from build123d import *

# Parameters (mm, degrees)
BOSS_EXTRUDE1_DEPTH = 10
SKETCH2_R           = 10.45
CUT_EXTRUDE1_DEPTH  = 7
SKETCH3_R           = 6.5
CUT_EXTRUDE2_DEPTH  = 24.087280048


with BuildPart() as part:
    # Sketch1 → Boss-Extrude1 (new body)
    with BuildSketch(Plane.YZ):
        with BuildLine():
            Line((-12.65, 0), (-12.65, 18))
            Line((-12.65, 18), (12.65, 18))
            Line((12.65, 18), (12.65, 0))
            ThreePointArc((12.65, 0), (0, -12.65), (-12.65, 0))
        make_face()
    extrude(amount=BOSS_EXTRUDE1_DEPTH)

    # Sketch2 → Cut-Extrude1 (cut)
    with BuildSketch(Plane.YZ.offset(10)):
        with Locations(Location((0, 0, 0), (0, 0, 270))):
            Circle(SKETCH2_R)
    extrude(amount=-CUT_EXTRUDE1_DEPTH, mode=Mode.SUBTRACT)

    # Sketch3 → Cut-Extrude2 (cut, through all)
    with BuildSketch(Plane.YZ.offset(3)):
        with Locations(Location((0, 0, 0), (0, 0, 270))):
            Circle(SKETCH3_R)
    extrude(amount=-CUT_EXTRUDE2_DEPTH, mode=Mode.SUBTRACT)


solid = part.part
The listing builds one solid part. Answer for the finished solid, in the listing's coordinates (mm). A direction names the side the tool comes from. Give positions to 0.01 mm unless a question says otherwise; leave off trailing zeros. Write each loop counter-clockwise with the first axis right and the second up, starting at its lowest first coordinate (ties: lowest second). Pieces come first, ordered by that corner, then holes.
Item 1: Which of the six approach directions +Z, -Z, +X, -X, +Y, -Y give full straight-line access (tool end or side, diameter ignored) to faces 5 (the flat face through (10, 6, 10)), 6 (the cylindrical face through (6.549, 3.139, -9.967))?
Item 2: Determine the mould class of faces 1 (the cylindrical face through (1.521, -3.955, 5.158)), 2 (the cylindrical face through (4.93, 0.278, -12.647)), 3 (the flat face through (5, -12.65, 9)), 4 (the flat face through (3, 0, -7)) for opening direction Z: released by +Z, released by -Z, zero draft, split by the parting line, or undercut.
Item 3: Find the intervals of material crossed by line 1 along Y through (x, z) = (7, 0); line 2 along Y through (x, z) = (2.45, 0); line 3 along Z through (x, y) = (7.5, 4.25), in increasing order.
Item 4: Section C-C, the plane x = 9 is taken. Write down the section's boundary in (y, z), plus the area to 3 significant figures.
Item 5: Flat-ended cylindrical pins translate along their axes: P1, Ø4, axis at y = 2.5, z = -2.5, coming from the +X side; P2, Ø6.5, axis at y = 2, z = 3, coming from the +X side; P3, Ø3, axis at x = 7.5, y = -8.5, coming from the -Z side; P4, Ø3, axis at x = 2.5, z = -3, coming from the -Y side. Find the tip coordinate at first contact, or state that the pin passes through.
Item 6: Section B-B, the plane z = 5.5 is taken. Write down the section's boundary in (x, y).
Item 7: Section D-D, the plane z = -7.5 is taken. Write down the section's boundary in (x, y).
Item 8: Section A-A, the plane y = 0 is taken. Write down the section's boundary in (x, z).
Completed:
1. face 5: +Z, -Z, +X, +Y, -Y
1. face 6: +X
2. face 1: undercut
2. face 2: released by -Z
2. face 3: zero draft
2. face 4: undercut
3. line 1: y = -12.65 to -10.45, 10.45 to 12.65
3. line 2: y = -12.65 to -6.5, 6.5 to 12.65
3. line 3: z = -11.91 to -9.55, 9.55 to 18
4. outline: (-12.65, 0) arc R12.65 ccw to (12.65, 0) - (12.65, 18) - (-12.65, 18) - close; hole circle Ø20.9 at (0, 0)
4. area: 364 mm2
5. P1: passes through
5. P2: stops at x = 3
5. P3: stops at z = -10.54
5. P4: stops at y = -12.56
6. outline: (0, -12.65) - (10, -12.65) - (10, -8.89) - (3, -8.89) - (3, -3.46) - (0, -3.46) - close; (0, 3.46) - (3, 3.46) - (3, 8.89) - (10, 8.89) - (10, 12.65) - (0, 12.65) - close
7. outline: (0, -10.19) - (10, -10.19) - (10, -7.28) - (3, -7.28) - (3, 7.28) - (10, 7.28) - (10, 10.19) - (0, 10.19) - close
8. outline: (0, -12.65) - (10, -12.65) - (10, -10.45) - (3, -10.45) - (3, -6.5) - (0, -6.5) - close; (0, 6.5) - (3, 6.5) - (3, 10.45) - (10, 10.45) - (10, 18) - (0, 18) - close
